The listing builds one solid part. Answer for the finished solid, in the listing's coordinates (mm). Face numbers are marked on the shaded views. A direction names the side the tool comes from. Round coordinates to 2 decimals unless told otherwise and drop trailing zeros. Loops run counter-clockwise (first coordinate to the right, second up) from the corner with the lowest first, then second, coordinate; pieces in that order, holes last. Notation, with made-up numbers: M 3.5,-33 L 9.5,-33 A11 ccw 9.5,-17 Z; hole C -19.75,82 d8. An arc over 180 degrees is marked long. Answer as a JSON object with one key per item and string values.
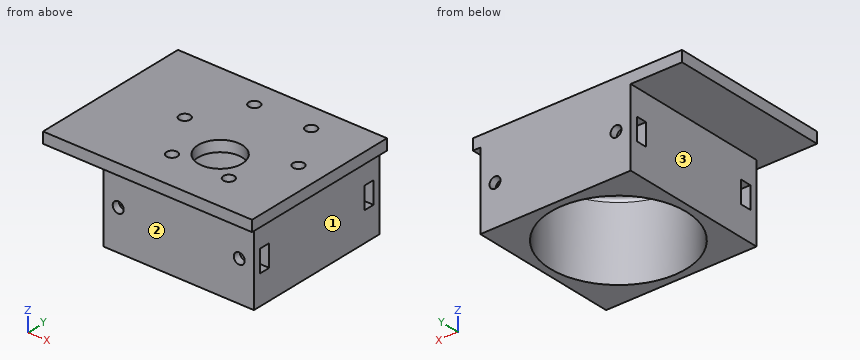
```python
from build123d import *

# Parameters (mm, degrees)
SKETCH_1_W             = 69
SKETCH_1_H             = 44
EXTRUDE_624_DEPTH      = 3
SKETCH_2_R             = 1.5
SKETCH_2_R_2           = 6
CUT_EXTRUDE_837_DEPTH  = 3
SKETCH_4_R             = 20.5
SKETCH_4_R_2           = 18.5
EXTRUDE_1079_DEPTH     = 21
EXTRUDE_1525_DEPTH     = 21
SKETCH_20_W            = 1.345299462
SKETCH_20_H            = 6
CUT_EXTRUDE_2290_DEPTH = 3
SKETCH_21_W            = 1.345299462
SKETCH_21_H            = 6
CUT_EXTRUDE_2993_DEPTH = 3
SKETCH_11_W            = 41
SKETCH_11_H            = 2
EXTRUDE_3369_DEPTH     = 21
SKETCH_16_R            = 1.5
CUT_EXTRUDE_3664_DEPTH = 6.5
SKETCH_17_R            = 1.5
CUT_EXTRUDE_4007_DEPTH = 6.5
SKETCH_22_W            = 12
SKETCH_22_H            = 44
CUT_EXTRUDE_4241_DEPTH = 3
FILLET_1_R             = 1


with BuildPart() as part:
    # 草图1 → Extrude 624 (new body)
    with BuildSketch(Plane.XY):
        with Locations((0, -1.5)):
            Rectangle(SKETCH_1_W, SKETCH_1_H)
    extrude(amount=EXTRUDE_624_DEPTH)

    # 草图2 → Cut-Extrude 837 (cut)
    with BuildSketch(Plane(origin=(0, 0, 0), x_dir=(-1, 0, 0), z_dir=(0, 0, -1))):
        with Locations((-15.5, 0)):
            Circle(SKETCH_2_R)
        with Locations((-7.75, 13.423393759)):
            Circle(SKETCH_2_R)
        with Locations((7.75, 13.423393759)):
            Circle(SKETCH_2_R)
        with Locations((15.5, 0)):
            Circle(SKETCH_2_R)
        with Locations((7.75, -13.423393759)):
            Circle(SKETCH_2_R)
        with Locations((-7.75, -13.423393759)):
            Circle(SKETCH_2_R)
        with Locations((0, -7)):
            Circle(SKETCH_2_R_2)
    extrude(amount=-CUT_EXTRUDE_837_DEPTH, mode=Mode.SUBTRACT)

    # 草图4 → Extrude 1079 (add)
    with BuildSketch(Plane(origin=(0, 0, 0), x_dir=(-1, 0, 0), z_dir=(0, 0, -1))):
        Circle(SKETCH_4_R)
        Circle(SKETCH_4_R_2, mode=Mode.SUBTRACT)
    extrude(amount=EXTRUDE_1079_DEPTH)

    # 草图13 → Extrude 1525 (add)
    with BuildSketch(Plane(origin=(0, 0, 0), x_dir=(-1, 0, 0), z_dir=(0, 0, -1))):
        with BuildLine():
            Line((-20.5, 18.5), (-20.5, -3.7e-08))
            ThreePointArc((-20.5, -3.7e-08), (-17.339277644, 10.936153381), (-8.831760866, 18.5))
            Line((-8.831760866, 18.5), (-20.5, 18.5))
        make_face()
        with BuildLine():
            Line((-20.5, -18.5), (-8.831760866, -18.5))
            ThreePointArc((-8.831760866, -18.5), (-17.339277624, -10.936153413), (-20.5, -3.7e-08))
            Line((-20.5, -3.7e-08), (-20.5, -18.5))
        make_face()
        with BuildLine():
            Line((8.831760866, -18.5), (20.5, -18.5))
            Line((20.5, -18.5), (20.5, 0))
            ThreePointArc((20.5, 0), (17.339277634, -10.936153397), (8.831760866, -18.5))
        make_face()
        with BuildLine():
            ThreePointArc((8.831760866, 18.5), (17.339277634, 10.936153397), (20.5, 0))
            Line((20.5, 0), (20.5, 18.5))
            Line((20.5, 18.5), (8.831760866, 18.5))
        make_face()
    extrude(amount=EXTRUDE_1525_DEPTH)

    # 草图20 → Cut-Extrude 2290 (cut)
    with BuildSketch(Plane.XZ.offset(18.5)):
        Polygon((19.154700538, -11.401923789), (19.154700538, -7), (18.232050808, -7), (14.767949192, -7), (13.035898385, -10), (14.767949192, -13), (19.154700538, -13), align=None)
        Polygon((20.5, -7), (19.154700538, -7), (19.154700538, -11.401923789), (20.5, -9.07179677), align=None)
        Polygon((20.5, -9.07179677), (19.154700538, -11.401923789), (19.154700538, -13), (20.5, -13), align=None)
        with Locations((-19.827350269, -10)):
            Rectangle(SKETCH_20_W, SKETCH_20_H)
        Polygon((-14.767949192, -7), (-19.154700538, -7), (-19.154700538, -13), (-14.767949192, -13), (-13.035898385, -10), align=None)
    extrude(amount=-CUT_EXTRUDE_2290_DEPTH, mode=Mode.SUBTRACT)

    # 草图21 → Cut-Extrude 2993 (cut)
    with BuildSketch(Plane(origin=(0, 18.5, 0), x_dir=(1, 0, 0), z_dir=(0, 1, 0))):
        Polygon((19.154700538, 8.598076211), (19.154700538, 13), (18.232050808, 13), (14.767949192, 13), (13.035898385, 10), (14.767949192, 7), (19.154700538, 7), align=None)
        Polygon((20.5, 13), (19.154700538, 13), (19.154700538, 8.598076211), (20.5, 10.92820323), align=None)
        Polygon((20.5, 10.92820323), (19.154700538, 8.598076211), (19.154700538, 7), (20.5, 7), align=None)
        with Locations((-19.827350269, 10)):
            Rectangle(SKETCH_21_W, SKETCH_21_H)
        Polygon((-14.767949192, 13), (-19.154700538, 13), (-19.154700538, 7), (-14.767949192, 7), (-13.035898385, 10), align=None)
    extrude(amount=-CUT_EXTRUDE_2993_DEPTH, mode=Mode.SUBTRACT)

    # 草图11 → Extrude 3369 (add)
    with BuildSketch(Plane(origin=(0, 0, 0), x_dir=(-1, 0, 0), z_dir=(0, 0, -1))):
        with Locations((0, 19.5)):
            Rectangle(SKETCH_11_W, SKETCH_11_H)
        with Locations((0, -19.5)):
            Rectangle(SKETCH_11_W, SKETCH_11_H)
    extrude(amount=EXTRUDE_3369_DEPTH)

    # 草图16 → Cut-Extrude 3664 (cut)
    with BuildSketch(Plane.XZ.offset(20.5)):
        with Locations((-16.5, -10)):
            Circle(SKETCH_16_R)
        with Locations((16.5, -10)):
            Circle(SKETCH_16_R)
    extrude(amount=-CUT_EXTRUDE_3664_DEPTH, mode=Mode.SUBTRACT)

    # 草图17 → Cut-Extrude 4007 (cut)
    with BuildSketch(Plane(origin=(0, 20.5, 0), x_dir=(1, 0, 0), z_dir=(0, 1, 0))):
        with Locations((-16.5, 10)):
            Circle(SKETCH_17_R)
        with Locations((16.5, 10)):
            Circle(SKETCH_17_R)
    extrude(amount=-CUT_EXTRUDE_4007_DEPTH, mode=Mode.SUBTRACT)

    # 草图22 → Cut-Extrude 4241 (cut)
    with BuildSketch(Plane(origin=(0, 0, 0), x_dir=(-1, 0, 0), z_dir=(0, 0, -1))):
        with Locations((-28.5, -1.5)):
            Rectangle(SKETCH_22_W, SKETCH_22_H)
    extrude(amount=-CUT_EXTRUDE_4241_DEPTH, mode=Mode.SUBTRACT)

    # 圆角1
    fillet_1_edges = [part.edges().sort_by_distance(p)[0] for p in [
        (18.5, 0, 0),
    ]]
    fillet(fillet_1_edges, radius=FILLET_1_R)


solid = part.part
```
Item 1: The part is cut by section A-A (x = -19.5). Give the vertices of the cut face in (y, z), then the cut area to 3 significant figures.
Values follow:
{"outline": "M -23.5,0 L -20.5,0 L -20.5,-21 L 20.5,-21 L 20.5,3 L -23.5,3 Z; hole M -18.5,-13 L -15.5,-13 L -15.5,-7 L -18.5,-7 Z; hole M 15.5,-13 L 18.5,-13 L 18.5,-7 L 15.5,-7 Z", "area": "957 mm^2"}
Item 2: Flat-ended cylindrical pins translate along their axes: P1, Ø10, axis at y = 2, z = -10.5, coming from the +X side; P2, Ø2.5, axis at x = -16.5, z = -10, coming from the -Y side; P3, Ø2, axis at x = -20, z = -10, coming from the -Y side. Find the tip coordinate at first contact, or state that the pin passes through.
Values follow:
{"P1": "x = 20.5", "P2": "y = -14", "P3": "y = -20.5"}
Item 3: Straight lines are drawn through the part: line 1 (X direction, y = 19.85, z = -10); line 2 (Y direction, x = 7.75, z = 1); line 3 (Z direction, x = -17, y = -16.5). For each, find the intervals that lie inside material, in ascending order.
Values follow:
{"line 1": "-20.5 to -18, -15 to 15, 18 to 20.5", "line 2": "-23.5 to -14.92, -11.92 to 11.92, 14.92 to 20.5", "line 3": "-21 to -13, -7 to 3"}
Item 4: The part is cut by section B-B (z = -14). Give the vertices of the cut face in (x, y), then the cut area to 3 significant figures.
Values follow:
{"outline": "M -20.5,-20.5 L 20.5,-20.5 L 20.5,20.5 L -20.5,20.5 Z; hole C 0,0 d37", "area": "606 mm^2"}
Item 5: The part is cut by section C-C (x = -29). Give the vertices of the cut face in (y, z).
Values follow:
{"outline": "M -23.5,0 L 20.5,0 L 20.5,3 L -23.5,3 Z"}
Item 6: The part is cut by section D-D (x = -7.75). Give the number of separate pieces and of enclosed holes in the cut face, then the cut area to 3 significant figures.
Values follow:
{"separate pieces": "3", "enclosed holes": "0", "area": "270 mm^2"}
Item 7: Which of the six approach directions +Z, -Z, +X, -X, +Y, -Y give full straight-line access (tool end or side, diameter ignored) to the marked faces 1, 2 and 3?
Values follow:
{"face 1": "-Z, +X, +Y, -Y", "face 2": "-Z, +X, -X, -Y", "face 3": "-Z, -X, +Y, -Y"}
